Here's how the part is built. I have some questions about the finished solid (model axes, mm). Face numbers are marked on the shaded views. A direction names the side the tool comes from. Coordinates: 2 decimals unless noted, no trailing zeros. Loops run counter-clockwise (first coordinate to the right, second up) from the corner with the lowest first, then second, coordinate; pieces in that order, holes last. Notation, with made-up numbers: (16, 77) -> (27, 77) arc R10 cw to (27, 86) -> close; hole circle Ø1 at (83, 62.5). An arc over 180 degrees is marked (long way). Answer as a JSON object with one key per item and string values. Group by question number.
1) I need wall thicknesses on probe 1 along Y at (x, z) = (33.5, 12); probe 2 along Y at (x, z) = (-23.5, 19.5); probe 3 along X at (y, z) = (13.75, 1) (3 decimals). Which ranges of each line are inside material? Lowest first, please. Write a range as [from, to].
2) I want a section at D-D (x = 30). Write out the boundary of the cut face in (y, z) (3 decimals), then the cut area to 3 significant figures.
3) Which directions (+Z, -Z, +X, -X, +Y, -Y) give clear straight access to the entire face, cutting with the end or side of a thin tool? Please do the marked faces 1 and 2.
4) I want a section at B-B (x = -30.5). Write out the boundary of the cut face in (y, z) (3 decimals), then the cut area to 3 significant figures.
5) I want a section at C-C (z = -14.5). Write out the boundary of the cut face in (x, y) (3 decimals), then the cut area to 3 significant figures.
6) I'm going to push flat-ended pins straight in: pin 1 (0.5 mm diameter, centred on x = -37.5, y = 12.5, fed in from +Z) (3 decimals); pin 2 (1.8 mm diameter, centred on y = 13.5, z = -19, fed in from +X) (3 decimals); pin 3 (17.5 mm diameter, centred on x = -38, z = 20.5, fed in from +Y). Where does each tip first touch, or does it pass through?
7) I want a section at A-A (y = 12.75). Write out the boundary of the cut face in (x, z) (3 decimals), then the cut area to 3 significant figures.
Autodesk Inventor part; units mm, degrees
ref_plane "YZ Plane" through (0, 0, 0) normal (1, 0, 0) x (0, 1, 0)
ref_plane "XZ Plane" through (0, 0, 0) normal (0, 1, 0) x (-1, 0, 0)
ref_plane "XY Plane" through (0, 0, 0) normal (0, 0, 1) x (1, 0, 0)
sketch "Sketch1" plane through (0, 0, 0) normal (0, 1, 0) x (-1, 0, 0)
  line L0 (43.575, 28.025) -> (-43.575, 28.025)
  line L1 (-43.575, 28.025) -> (-43.575, -27.975)
  line L2 (-43.575, -27.975) -> (43.575, -27.975)
  line L3 (43.575, -27.975) -> (43.575, 28.025)
  point P0 (0, 0)
  dimension "d0" = 87.15
  dimension "d1" = 56
  dimension "d2" = 27.975
  dimension "d3" = 43.575
extrude "Extrusion1" add sketch "Sketch1" along normal blind 11.8
sketch "Sketch4" plane through (0, 11.8, 0) normal (0, 1, 0) x (1, 0, 0)
  line L0 (-43.575, 25.725) -> (-25.825, 25.725)
  line L1 (-25.825, 25.725) -> (-25.825, 12.725)
  line L2 (-25.825, 12.725) -> (-43.575, 12.725)
  line L3 (-43.575, 12.725) -> (-43.575, 25.725)
  line L4 (-43.575, 7.725) -> (-25.825, 7.725)
  line L5 (-25.825, 7.725) -> (-25.825, -5.275)
  line L6 (-25.825, -5.275) -> (-43.575, -5.275)
  line L7 (-43.575, -5.275) -> (-43.575, 7.725)
  line L8 (43.575, 27.975) -> (-43.575, 27.975)
  line L9 (-43.575, 27.975) -> (-43.575, -28.025)
  point P0 (0, 0)
  dimension "d12" = 17.75
  dimension "d13" = 13
  dimension "d14" = 5
  dimension "d15" = 13
  dimension "d16" = 17.75
  dimension "d43" = 2.25
extrude "Extrusion2" add sketch "Sketch4" along normal blind 3.7
sketch "Sketch6" plane through (0, 11.8, 0) normal (0, 1, 0) x (1, 0, 0)
  line L0 (-43.575, -9.775) -> (-22.275, -9.775)
  line L1 (-22.275, -9.775) -> (-22.275, -25.775)
  line L2 (-22.275, -25.775) -> (-43.575, -25.775)
  line L3 (-43.575, -25.775) -> (-43.575, -9.775)
  line L4 (-43.575, 25.725) -> (-25.825, 25.725)
  line L5 (-43.575, 27.975) -> (-43.575, 25.725)
  line L6 (-43.575, -5.275) -> (-25.825, -5.275)
  point P0 (0, 0)
  dimension "d19" = 16
  dimension "d20" = 21.3
  dimension "d22" = 0
  dimension "d44" = 4.5
extrude "Extrusion3" add sketch "Sketch6" along normal blind 1.8
sketch "Sketch10" plane through (43.575, 0, 28.025) normal (1, 0, 0) x (0, 0, -1)
  point P0 (28.025, 0)
sketch "Sketch11" plane through (0, 11.8, 0) normal (0, 1, 0) x (1, 0, 0)
  circle A0 centre (-18.425, -24.525) radius 1.5
  circle A1 centre (-18.425, 24.475) radius 1.5
  circle A2 centre (40.075, -24.525) radius 1.5
  circle A3 centre (40.075, 24.475) radius 1.5
  line L0 (-43.575, -5.275) -> (-43.575, -9.775)
  line L1 (-43.575, 27.975) -> (-43.575, 25.725)
  line L2 (-43.575, -28.025) -> (43.575, -28.025)
  line L3 (43.575, -28.025) -> (43.575, 27.975)
  line L4 (43.575, 27.975) -> (-43.575, 27.975)
  point P0 (0, 0)
  dimension "d45" = 3
  dimension "d46" = 3
  dimension "d47" = 3
  dimension "d48" = 3
  dimension "d50" = 58.5
  dimension "d51" = 58.5
  dimension "d55" = 3.5
  dimension "d56" = 3.5
  dimension "d59" = 3.5
  dimension "d60" = 3.5
  dimension "d61" = 3.5
  dimension "d62" = 3.5
extrude "Extrusion7" cut sketch "Sketch11" against normal through all
properties part number "RaspPi_Model"
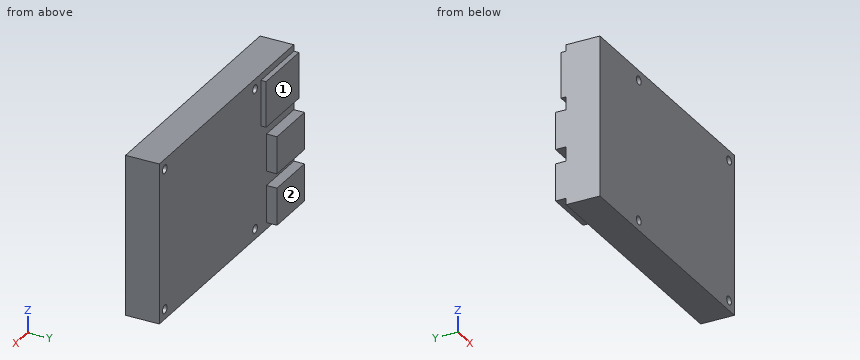
Determined:
{
 "1": {"probe 1": "[0, 11.8]", "probe 2": "[0, 13.6]", "probe 3": "[-43.575, -25.825]"},
 "2": {"outline": "(0, -27.975) -> (11.8, -27.975) -> (11.8, 28.025) -> (0, 28.025) -> close", "area": "661 mm^2"},
 "3": {"face 1": "+Z, +X, -X, +Y", "face 2": "+Z, -Z, +X, -X, +Y"},
 "4": {"outline": "(0, -27.975) -> (11.8, -27.975) -> (11.8, -25.725) -> (15.5, -25.725) -> (15.5, -12.725) -> (11.8, -12.725) -> (11.8, -7.725) -> (15.5, -7.725) -> (15.5, 5.275) -> (11.8, 5.275) -> (11.8, 9.775) -> (13.6, 9.775) -> (13.6, 25.775) -> (11.8, 25.775) -> (11.8, 28.025) -> (0, 28.025) -> close", "area": "786 mm^2"},
 "5": {"outline": "(-43.575, 0) -> (43.575, 0) -> (43.575, 11.8) -> (-25.825, 11.8) -> (-25.825, 15.5) -> (-43.575, 15.5) -> close", "area": "1,090 mm^2"},
 "6": {"pin 1": "z = 25.775", "pin 2": "x = -25.825", "pin 3": "y = 13.6"},
 "7": {"outline": "(-43.575, -25.725) -> (-25.825, -25.725) -> (-25.825, -12.725) -> (-43.575, -12.725) -> close; (-43.575, -7.725) -> (-25.825, -7.725) -> (-25.825, 5.275) -> (-43.575, 5.275) -> close; (-43.575, 9.775) -> (-22.275, 9.775) -> (-22.275, 25.775) -> (-43.575, 25.775) -> close", "area": "802 mm^2"}
}
